```python
from build123d import *

# Parameters (mm, degrees)
F1_DEPTH = 10
F2_DEPTH = 5
F3_W     = 4.9271763038
F3_H     = 2
F4_DEPTH = 5
F6_DEPTH = 4.9271763038
F7_DEPTH = 0.2
F8_DEPTH = 0.2


with BuildPart() as f1:
    # F0 (on Top) → F1 (new body)
    with BuildSketch(Plane.XY):
        with BuildLine():
            Line((-35, -15), (5, -15))
            ThreePointArc((5, -15), (13.7867965644, 6.2132034356), (35, 15))
            Line((35, 15), (-35, 15))
            Line((-35, 15), (-35, -15))
        make_face()
    extrude(amount=F1_DEPTH)

    # F0 (on Top) → F2 (join)
    with BuildSketch(Plane.XY):
        with BuildLine():
            Line((5, -15), (7.5, -15))
            ThreePointArc((7.5, -15), (15.5545635174, 4.4454364826), (35, 12.5))
            Line((35, 12.5), (35, 15))
            ThreePointArc((35, 15), (13.7867965644, 6.2132034356), (5, -15))
        make_face()
        with BuildLine():
            Line((7.5, -15), (12.5, -15))
            ThreePointArc((12.5, -15), (19.0900974233, 0.9099025767), (35, 7.5))
            Line((35, 7.5), (35, 12.5))
            ThreePointArc((35, 12.5), (15.5545635174, 4.4454364826), (7.5, -15))
        make_face()
        with BuildLine():
            ThreePointArc((62.5, -15), (35, -42.5), (7.5, -15))
            Line((7.5, -15), (5, -15))
            ThreePointArc((5, -15), (35, -45), (65, -15))
            ThreePointArc((65, -15), (56.2132034356, 6.2132034356), (35, 15))
            Line((35, 15), (35, 12.5))
            ThreePointArc((35, 12.5), (54.4454364826, 4.4454364826), (62.5, -15))
        make_face()
        with BuildLine():
            ThreePointArc((57.5, -15), (35, -37.5), (12.5, -15))
            Line((12.5, -15), (7.5, -15))
            ThreePointArc((7.5, -15), (35, -42.5), (62.5, -15))
            ThreePointArc((62.5, -15), (54.4454364826, 4.4454364826), (35, 12.5))
            Line((35, 12.5), (35, 7.5))
            ThreePointArc((35, 7.5), (50.9099025767, 0.9099025767), (57.5, -15))
        make_face()
        with BuildLine():
            Line((12.5, -15), (32.5, -15))
            ThreePointArc((32.5, -15), (33.232233047, -13.232233047), (35, -12.5))
            Line((35, -12.5), (35, 7.5))
            ThreePointArc((35, 7.5), (19.0900974233, 0.9099025767), (12.5, -15))
        make_face()
        with BuildLine():
            ThreePointArc((37.5, -15), (35, -17.5), (32.5, -15))
            Line((32.5, -15), (12.5, -15))
            ThreePointArc((12.5, -15), (35, -37.5), (57.5, -15))
            ThreePointArc((57.5, -15), (50.9099025767, 0.9099025767), (35, 7.5))
            Line((35, 7.5), (35, -12.5))
            ThreePointArc((35, -12.5), (36.767766953, -13.232233047), (37.5, -15))
        make_face()
    extrude(amount=F2_DEPTH)

    # F3 (on face) → F4 (join, through all)
    with BuildSketch(Plane.XY.offset(5)):
        with Locations((59.9635881519, -14)):
            Rectangle(F3_W, F3_H)
        with Locations((59.9635881519, -16)):
            Rectangle(F3_W, F3_H)
    extrude(amount=F4_DEPTH)

    # F5 (on face) → F6 (cut, through all)
    with BuildSketch(Plane.YZ.offset(62.4271763038)):
        Polygon((-17, 10), (-17, 5), (-15, 10), align=None)
        Polygon((-13, 10), (-15, 10), (-13, 5), align=None)
    extrude(amount=-F6_DEPTH, mode=Mode.SUBTRACT)

    # F7 (cut): a face of the model
    f7_faces = [f1.faces().sort_by_distance(p)[0] for p in [
        (62.4271763038, -15, 6.6666666667),
    ]]
    extrude(f7_faces, amount=F7_DEPTH, mode=Mode.SUBTRACT)

    # F8 (cut): a face of the model
    f8_faces = [f1.faces().sort_by_distance(p)[0] for p in [
        (57.5, -15, 6.6666666667),
    ]]
    extrude(f8_faces, amount=-F8_DEPTH, mode=Mode.SUBTRACT)


solid = f1.part
```
Check sheet for the modelled part. Datum: model origin and axes. Units: mm. A direction names the side the tool comes from. Coordinates: 2 decimals unless noted, no trailing zeros. Loops run counter-clockwise (first coordinate to the right, second up) from the corner with the lowest first, then second, coordinate; pieces in that order, holes last. Notation, with made-up numbers: M 78.5,22 L 103.5,22 A22 cw 103.5,41 Z; hole C -35.5,42.25 d6. An arc over 180 degrees is marked long. Answer as a JSON object with one key per item and string values.
1. Sectioned sample at C-C on y = 2.5. Record the cut outline in (x, z).
Outcome:
{"outline": "M -35,0 L 59.37,0 L 59.37,5 L 10.63,5 L 10.63,10 L -35,10 Z"}
2. Sectioned sample at D-D on x = 1.5. Record the cut outline in (y, z).
Outcome:
{"outline": "M -15,0 L 15,0 L 15,10 L -15,10 Z"}
3. Scan lines: L1, parallel to Y at x = -28, z = 2.5; L2, parallel to Z at x = 36, y = -17.5; L3, parallel to X at y = -19.5, z = 3.5. Record each from-to range of solid material in increasing order. Write a range as from..to.
Outcome:
{"L1": "-15..15", "L2": "0..5", "L3": "5.34..64.66"}
4. Access from +Z, -Z, +X, -X, +Y, -Y to the whole of each face (thin tool, end or side, straight path). Record for faces 1 (the flat face through (60.1, -14, 7.5)), 2 (the flat face through (62.427, -15, 7)), 3 (the flat face through (-15, -15, 5)), 4 (the flat face through (57.7, -15, 7)).
Outcome:
{"face 1": "+Z, +X, +Y", "face 2": "+Z, +X, +Y, -Y", "face 3": "+Z, -Z, -X, -Y", "face 4": "+Z, +Y, -Y"}
5. Depth check by flat-ended pin: P1, Ø3, axis at x = -11, z = 2.5, coming from the -Y side; P2, Ø1, axis at y = -18.5, z = 7.5, coming from the -X side; P3, Ø5, axis at x = 31.5, y = -17, coming from the +Z side; P4, Ø2, axis at y = -15, z = 7, coming from the +X side. Enter the tip coordinate at first touch or a pass-through.
Outcome:
{"P1": "y = -15", "P2": "through", "P3": "z = 5", "P4": "x = 62.43"}
6. Sectioned sample at A-A on z = 8.25. Record the cut outline in (x, y).
Outcome:
{"outline": "M -35,-15 L 5,-15 A30 cw 35,15 L -35,15 Z; M 57.7,-15.7 L 62.43,-15.7 L 62.43,-14.3 L 57.7,-14.3 Z"}
